from build123d import *

# Parameters (mm, degrees)
F0_W      = 61.976
F0_H      = 133.096
F1_DEPTH  = 7.62
F2_DEPTH  = 0.254
F3_R      = 7.62
F4_R      = 5.08
F6_DEPTH  = 0.254
F7_W      = 26.6171786934
F7_H      = 2.5910458062
F7_W_2    = 12.6955425367
F8_DEPTH  = 381
F9_W      = 12.6955425367
F9_H      = 2.5910458062
F10_DEPTH = 2.54
F11_W     = 13.3085893467
F11_H     = 2.5910458062
F12_DEPTH = 2.54
F13_W     = 22.86
F13_H     = 12.7
F14_DEPTH = 25.4
F15_R     = 2.54
F16_W     = 12.7
F16_H     = 5.08
F17_DEPTH = 25.4
F18_R     = 1.27
F19_W     = 19.05
F19_H     = 3.81
F20_DEPTH = 25.4
F21_W     = 10.6675168499
F21_H     = 3.81
F22_DEPTH = 25.4


with BuildPart() as f1:
    # F0 (on Top) → F1 (new body)
    with BuildSketch(Plane.XY):
        Polygon((-33.528, 0), (0, 0), (33.528, 0), (33.528, 138.176), (0, 138.176), (-33.528, 138.176), align=None)
        with Locations((0, 69.088)):
            Rectangle(F0_W, F0_H, mode=Mode.SUBTRACT)
    extrude(amount=F1_DEPTH)

    # F0 (on Top) → F2 (join)
    with BuildSketch(Plane.XY):
        with Locations((0, 69.088)):
            Rectangle(F0_W, F0_H)
    extrude(amount=F2_DEPTH)

    # F3
    f3_edges = [f1.edges().sort_by_distance(p)[0] for p in [
        (-33.528, 0, 3.81),
        (33.528, 0, 3.81),
        (33.528, 138.176, 3.81),
        (-33.528, 138.176, 3.81),
    ]]
    fillet(f3_edges, radius=F3_R)

    # F4
    f4_edges = [f1.edges().sort_by_distance(p)[0] for p in [
        (-30.988, 135.636, 3.937),
        (30.988, 135.636, 3.937),
        (-30.988, 2.54, 3.937),
        (30.988, 2.54, 3.937),
    ]]
    fillet(f4_edges, radius=F4_R)

    # F5 (on face) → F6 (join)
    with BuildSketch(Plane.XY):
        Polygon((-30.988, 58.8372340277), (-33.528, 56.507691741), (-30.988, 56.507691741), align=None)
        Polygon((16.764, 69.088), (0, 69.088), (-16.764, 69.088), (-16.764, 61.135802418), (-28.4817721695, 61.135802418), (-30.988, 58.8372340277), (-30.988, 56.507691741), (-16.764, 56.507691741), (-16.764, 52.1295331419), (-26.285154745, 52.1295331419), (-30.988, 46.9043472506), (-30.988, 44.0822318196), (0, 44.0822318196), (30.988, 44.0822318196), (30.988, 47.1902959351), (26.9515123218, 52.1295331419), (0, 52.1295331419), (0, 61.135802418), (24.7533507645, 61.135802418), align=None)
        Polygon((-16.764, 69.088), (0, 69.088), (-16.764, 102.7458906174), align=None)
        Polygon((-30.988, 46.9043472506), (-33.528, 44.0822318196), (-30.988, 44.0822318196), align=None)
    extrude(amount=-F6_DEPTH)

    # F7 (on face) → F8 (cut)
    with BuildSketch(Plane(origin=(-33.528, 0, 0), x_dir=(0, -1, 0), z_dir=(-1, 0, 0))):
        with Locations((-36.9863724336, 4.5639382442)):
            Rectangle(F7_W, F7_H)
        with Locations((-14.7045073099, 4.5639382442)):
            Rectangle(F7_W_2, F7_H)
    extrude(amount=-F8_DEPTH, mode=Mode.SUBTRACT)

    # F9 (on face) → F10 (join)
    with BuildSketch(Plane(origin=(-33.528, 0, 0), x_dir=(0, -1, 0), z_dir=(-1, 0, 0))):
        with Locations((-14.7045073099, 4.5639382442)):
            Rectangle(F9_W, F9_H)
    extrude(amount=-F10_DEPTH)

    # F11 (on face) → F12 (join)
    with BuildSketch(Plane(origin=(-33.528, 0, 0), x_dir=(0, -1, 0), z_dir=(-1, 0, 0))):
        with Locations((-43.640667107, 4.5639382442)):
            Rectangle(F11_W, F11_H)
    extrude(amount=-F12_DEPTH)

    # F13 (on face) → F14 (cut)
    with BuildSketch(Plane.XY):
        with Locations((-19.558, 8.89)):
            Rectangle(F13_W, F13_H)
    extrude(amount=F14_DEPTH, mode=Mode.SUBTRACT)

    # F15
    f15_edges = [f1.edges().sort_by_distance(p)[0] for p in [
        (-8.128, 15.24, 0.127),
        (-8.128, 2.54, 0.127),
        (-30.988, 2.54, 3.81),
        (-30.988, 15.24, 0.127),
    ]]
    fillet(f15_edges, radius=F15_R)

    # F16 (on face) → F17 (cut)
    with BuildSketch(Plane(origin=(0, 138.176, 0), x_dir=(-1, 0, 0), z_dir=(0, 1, 0))):
        with Locations((-19.558, 3.81)):
            Rectangle(F16_W, F16_H)
    extrude(amount=-F17_DEPTH, mode=Mode.SUBTRACT)

    # F18
    f18_edges = [f1.edges().sort_by_distance(p)[0] for p in [
        (13.208, 136.906, 1.27),
        (25.908, 136.906, 1.27),
        (25.908, 136.906, 6.35),
        (13.208, 136.906, 6.35),
    ]]
    fillet(f18_edges, radius=F18_R)

    # F19 (on face) → F20 (cut)
    with BuildSketch(Plane(origin=(0, 138.176, 0), x_dir=(-1, 0, 0), z_dir=(0, 1, 0))):
        with Locations((16.383, 3.81)):
            Rectangle(F19_W, F19_H)
    extrude(amount=-F20_DEPTH, mode=Mode.SUBTRACT)

    # F21 (on face) → F22 (cut)
    with BuildSketch(Plane(origin=(0, 138.176, 0), x_dir=(-1, 0, 0), z_dir=(0, 1, 0))):
        with Locations((-1.8188538961, 3.175)):
            Rectangle(F21_W, F21_H)
    extrude(amount=-F22_DEPTH, mode=Mode.SUBTRACT)


solid = f1.part
Input: part model. Units: mm. Frame: model coordinates. A direction names the side the tool comes from. Coordinates: 2 decimals unless noted, no trailing zeros. Order: outer loops, then holes, each group sorted by start corner. A loop starts at its lowest first (then second) coordinate and runs counter-clockwise, first axis right, second up. Notation, with made-up numbers: M -27,-39 L -9,-39 A10 ccw -9,-34 Z; hole C 32,43 d11. An arc over 180 degrees is marked long. Answer as CSV lines item,"result".
1. Material intervals for line 1 (X direction, y = 131, z = 5); line 2 (Y direction, x = 26, z = 4); line 3 (Y direction, x = -13.5, z = 2), sorted ascending. Write a range as from..to.
Reported:
line 1,"-33.52..-30.97, 30.97..33.52"
line 2,"0..2.54, 135.64..138.18"
line 3,"0..2.54"
2. First-contact query: P1, Ø1.5, axis at x = -11.5, y = 114, coming from the +Z side; P2, Ø3, axis at y = 137, z = 3.5, coming from the -X side; P3, Ø2, axis at x = 32, z = 4, coming from the +Y side. Flat tips, straight axial feed; report the tip coordinate or a pass-through.
Reported:
P1,"z = 0.25"
P2,"x = -31.71"
P3,"y = 136.22"
3. Section C-C (x = -22). Return the cut outline in (y, z) (3 decimals).
Reported:
outline,"M 0,0 L 2.54,0 L 2.54,7.62 L 0,7.62 Z; M 15.24,0 L 44.082,0 L 44.082,-0.254 L 52.13,-0.254 L 52.13,0 L 56.508,0 L 56.508,-0.254 L 61.136,-0.254 L 61.136,0 L 138.176,0 L 138.176,1.905 L 135.636,1.905 L 135.636,0.254 L 15.24,0.254 Z; M 135.636,5.715 L 138.176,5.715 L 138.176,7.62 L 135.636,7.62 Z"
4. Section A-A (x = 4.5). Return the cut outline in (y, z), then the cut area to 3 significant figures.
Reported:
outline,"M 0,0 L 44.08,0 L 44.08,-0.25 L 52.13,-0.25 L 52.13,0 L 61.14,0 L 61.14,-0.25 L 69.09,-0.25 L 69.09,0 L 138.18,0 L 138.18,1.27 L 135.64,1.27 L 135.64,0.25 L 2.54,0.25 L 2.54,7.62 L 0,7.62 Z; M 135.64,5.08 L 138.18,5.08 L 138.18,7.62 L 135.64,7.62 Z"
area,"66.9 mm2"
5. Section D-D (y = 71). Return the cut outline in (x, z).
Reported:
outline,"M -33.53,0 L -16.76,0 L -16.76,-0.25 L -0.95,-0.25 L -0.95,0 L 33.53,0 L 33.53,7.62 L 30.99,7.62 L 30.99,0.25 L -30.99,0.25 L -30.99,7.62 L -33.53,7.62 Z"
6. Pull-direction query (Y, two-part tool) for faces 1 (the flat face through (0.4, 138.176, 5.4)), 2 (the flat face through (2, 137, 5.08)), 3 (the flat face through (-30.988, 69, 4)); classes: released by +Y, released by -Y, zero draft, split by the parting line, or undercut.
Reported:
face 1,"released by +Y"
face 2,"zero draft"
face 3,"undercut"
7. Section B-B (y = 41). Return the cut outline in (x, z), then the cut area to 3 significant figures.
Reported:
outline,"M -33.53,0 L 33.53,0 L 33.53,3.27 L 30.99,3.27 L 30.99,0.25 L -30.99,0.25 L -30.99,7.62 L -33.53,7.62 Z; M 30.99,5.86 L 33.53,5.86 L 33.53,7.62 L 30.99,7.62 Z"
area,"47.9 mm2"
8. Access query for faces 4 (the flat face through (7.153, 137, 3)), 5 (the flat face through (-32, 30, 3.268)), 6 (the flat face through (0, 135.636, 6)). Directions: +Z, -Z, +X, -X, +Y, -Y. A direction counts if a zero-diameter tool reaches every point of the face in a straight line with its end or side. Return the directions, or none.
Reported:
face 4,"+Y"
face 5,"+X, -X"
face 6,"+Z"
